```python
from build123d import *

# Parameters (mm, degrees)
SKETCH2_W           = 18
SKETCH2_H           = 30
BOSS_EXTRUDE1_DEPTH = 211.341
SKETCH3_W           = 4
SKETCH3_H           = 24
CUT_EXTRUDE1_DEPTH  = 1000
SKETCH4_R           = 5
CUT_EXTRUDE2_DEPTH  = 25
CUT_EXTRUDE3_START  = -25
SKETCH5_R           = 5
CUT_EXTRUDE3_DEPTH  = 25


with BuildPart() as part:
    # Sketch2 → Boss-Extrude1 (new body)
    with BuildSketch(Plane.XY):
        with Locations((9, -15)):
            Rectangle(SKETCH2_W, SKETCH2_H)
    extrude(amount=-BOSS_EXTRUDE1_DEPTH)

    # Sketch3 → Cut-Extrude1 (cut)
    with BuildSketch(Plane.XY):
        with Locations((16, -15)):
            Rectangle(SKETCH3_W, SKETCH3_H)
    extrude(amount=-CUT_EXTRUDE1_DEPTH, mode=Mode.SUBTRACT)

    # Sketch4 → Cut-Extrude2 (cut)
    with BuildSketch(Plane.XY):
        with Locations((7, -15)):
            Circle(SKETCH4_R)
    extrude(amount=-CUT_EXTRUDE2_DEPTH, mode=Mode.SUBTRACT)

    # Sketch5 → Cut-Extrude3 (cut)
    with BuildSketch(Plane(origin=(0, 0, -211.341), x_dir=(-1, 0, 0), z_dir=(0, 0, -1)).offset(CUT_EXTRUDE3_START)):
        with Locations(Location((-7, -15, 0), (0, 0, 180))):
            Circle(SKETCH5_R)
    extrude(amount=CUT_EXTRUDE3_DEPTH, mode=Mode.SUBTRACT)


solid = part.part
```
The model under review builds one solid part; all positions refer to its coordinate system, in mm. A direction names the side the tool comes from. Round coordinates to 2 decimals unless told otherwise and drop trailing zeros. Write each loop counter-clockwise with the first axis right and the second up, starting at its lowest first coordinate (ties: lowest second). Pieces come first, ordered by that corner, then holes. Notation, with made-up numbers: M 22,15 L 33,15 A29 cw 33,40 Z; hole C -8.5,30.25 d5. An arc over 180 degrees is marked long. Use CSV: the item, a comma, the result in double quotes. Start each with the question number.
(1) We need section B-B, the plane x = 7. State the section outline as (y, z) points.
(2) The part is to be moulded in two halves that separate along X. For faces 1 (the face through (9.307, -19.436, -12.325)), 2 (the face through (14, -15, -104)), 3 (the face through (16, -27, -104)), 4 (the face through (7, -15, -25)), say which applies: +X half, -X half, draft (parallel to the pull), parting line (faces both ways), or undercut.
(3) We need section A-A, the plane z = -144.5. State the section outline as (x, y) points.
(4) Clearance check with flat-ended pins moving along their axes: P1, Ø2, axis at x = 13, z = -27.5, coming from the +Y side; P2, Ø3, axis at x = 6, y = -14, coming from the +Z side; P3, Ø12, axis at y = -16, z = -71.5, coming from the +X side; P4, Ø3, axis at x = 5, y = -13, coming from the -Z side. State where each tip first meets the part, or that it passes through.
(5) For line 1 along Y through (x, z) = (7, -194.75); line 2 along X through (y, z) = (-15, -196.5); line 3 along Y through (x, z) = (14.25, -40.5), list the stretches that pass through material, from the lowest coordinate up.
(6) We need section C-C, the plane y = -15. State the section outline as (x, z) points, then the cut area to 3 significant figures.
(7) Tool access review of faces 5 (the face through (9, 0, -104)), 6 (the face through (16, -3, -104)), 7 (the face through (5.92, -10.12, -198.67)): name each direction out of +Z, -Z, +X, -X, +Y, -Y from which nothing blocks a thin tool from reaching the whole face with its end or side.
Findings:
1,outline,"M -30,-211.34 L -20,-211.34 L -20,-186.34 L -10,-186.34 L -10,-211.34 L 0,-211.34 L 0,0 L -10,0 L -10,-25 L -20,-25 L -20,0 L -30,0 Z"
2,face 1,"undercut"
2,face 2,"+X half"
2,face 3,"draft"
2,face 4,"undercut"
3,outline,"M 0,-30 L 18,-30 L 18,-27 L 14,-27 L 14,-3 L 18,-3 L 18,0 L 0,0 Z"
4,P1,"y = 0"
4,P2,"z = -25"
4,P3,"x = 14"
4,P4,"z = -186.34"
5,line 1,"-30 to -20, -10 to 0"
5,line 2,"0 to 2, 12 to 14"
5,line 3,"-30 to -27, -3 to 0"
6,outline,"M 0,-211.34 L 2,-211.34 L 2,-186.34 L 12,-186.34 L 12,-211.34 L 14,-211.34 L 14,0 L 12,0 L 12,-25 L 2,-25 L 2,0 L 0,0 Z"
6,area,"2,460 mm^2"
7,face 5,"+Z, -Z, +X, -X, +Y"
7,face 6,"+Z, -Z, +X"
7,face 7,"-Z"
